Autodesk Inventor part; units mm, degrees
ref_plane "YZ Plane" through (0, 0, 0) normal (1, 0, 0) x (0, 1, 0)
ref_plane "XZ Plane" through (0, 0, 0) normal (0, 1, 0) x (-1, 0, 0)
ref_plane "XY Plane" through (0, 0, 0) normal (0, 0, 1) x (1, 0, 0)
sketch "Эскиз1" plane through (0, 0, 0) normal (0, 0, 1) x (1, 0, 0)
  line L0 (-16.05, 21) -> (16.05, 21)
  line L1 (16.05, 21) -> (16.05, -21)
  line L2 (16.05, -21) -> (-16.05, -21)
  line L3 (-16.05, -21) -> (-16.05, 21)
  point P0 (0, 0)
  point P1 (0, 21)
  point P2 (16.05, 0)
  dimension "d0" = 32.1
  dimension "d1" = 42
extrude "Выдавливание1" add sketch "Эскиз1" along normal blind 2.5
sketch "Эскиз2" plane through (0, 0, 0) normal (0, 1, 0) x (-1, 0, 0)
  line L0 (16.05, 0) -> (-16.05, 0) construction
  line L1 (16.05, 0) -> (16.05, 2.5) construction
  line L2 (-16.05, 2.5) -> (16.05, 2.5) construction
  line L3 (-16.05, 0) -> (-16.05, 2.5) construction
  line L4 (-13.75, 0) -> (-13.75, -3)
  line L5 (-13.75, -3) -> (-16.05, -3)
  line L6 (-16.05, -3) -> (-16.05, -1.8)
  line L7 (-16.05, -1.8) -> (-14.95, -1.8)
  line L8 (-14.95, -1.8) -> (-14.95, 0)
  line L9 (-14.95, 0) -> (-13.75, 0)
  line L10 (13.75, 0) -> (13.75, -3)
  line L11 (13.75, -3) -> (16.05, -3)
  line L12 (16.05, -3) -> (16.05, -1.8)
  line L13 (16.05, -1.8) -> (14.95, -1.8)
  line L14 (14.95, -1.8) -> (14.95, 0)
  line L15 (14.95, 0) -> (13.75, 0)
  point P0 (0, 0)
  dimension "d4" = 2.3
  dimension "d5" = 1.2
  dimension "d6" = 5.5
extrude "Выдавливание2" add sketch "Эскиз2" along normal mid plane 5.1
sketch "Эскиз3" plane through (0, 0, 2.5) normal (0, 0, 1) x (1, 0, 0)
  line L0 (17.05, 2.55) -> (14.95, 2.55)
  line L1 (14.95, 2.55) -> (14.95, -2.55)
  line L2 (14.95, -2.55) -> (17.05, -2.55)
  line L3 (17.05, -2.55) -> (17.05, 2.55)
  line L4 (-14.95, 2.55) -> (-17.05, 2.55)
  line L5 (-17.05, 2.55) -> (-17.05, -2.55)
  line L6 (-17.05, -2.55) -> (-14.95, -2.55)
  line L7 (-14.95, -2.55) -> (-14.95, 2.55)
  line L8 (-16.05, 21) -> (-16.05, -21) construction
  line L9 (16.05, -21) -> (16.05, 21) construction
  line L10 (16.05, -2.55) -> (16.05, 2.55) construction
  line L11 (14.95, 2.55) -> (16.05, 2.55) construction
  line L12 (14.95, -2.55) -> (14.95, 2.55) construction
  line L13 (16.05, -2.55) -> (14.95, -2.55) construction
  line L14 (-14.95, 2.55) -> (-14.95, -2.55) construction
  line L15 (-16.05, 2.55) -> (-14.95, 2.55) construction
  line L16 (-16.05, 2.55) -> (-16.05, -2.55) construction
  line L17 (-14.95, -2.55) -> (-16.05, -2.55) construction
  point P0 (0, 0)
  dimension "d9" = 1
  dimension "d10" = 1
extrude "Выдавливание3" cut sketch "Эскиз3" against normal up to surface (4.3 mm away)
sketch "Эскиз4" plane through (0, 0, 0) normal (0, 0, -1) x (-1, 0, 0)
  line L0 (13.75, -18.7) -> (-13.75, -18.7)
  line L1 (-13.75, -18.7) -> (-13.75, 18.7)
  line L2 (-13.75, 18.7) -> (13.75, 18.7)
  line L3 (13.75, 18.7) -> (13.75, -18.7)
  line L4 (-16.05, -21) -> (16.05, -21) construction
  line L5 (16.05, 21) -> (-16.05, 21) construction
  line L6 (13.75, -2.55) -> (13.75, 2.55) construction
  line L7 (-13.75, 2.55) -> (-13.75, -2.55) construction
  line L8 (16.05, -2.55) -> (16.05, -21) construction
  point P0 (0, 0)
  dimension "d13" = 2.3
  dimension "d14" = 2.3
  dimension "d15" = 2.3
extrude "Выдавливание4" cut sketch "Эскиз4" against normal blind 0.25
sketch "Эскиз5" plane through (0, 0, 2.5) normal (0, 0, 1) x (1, 0, 0)
  line L0 (14.95, 19.9) -> (-14.95, 19.9)
  line L1 (-14.95, 19.9) -> (-14.95, -19.9)
  line L2 (-14.95, -19.9) -> (14.95, -19.9)
  line L3 (14.95, -19.9) -> (14.95, 19.9)
  line L4 (14.95, -2.55) -> (14.95, 2.55) construction
  line L5 (-14.95, 2.55) -> (-14.95, -2.55) construction
  line L6 (16.05, 2.55) -> (16.05, 21) construction
  line L7 (16.05, 21) -> (-16.05, 21) construction
  line L8 (-16.05, -21) -> (16.05, -21) construction
  point P0 (0, 0)
  dimension "d18" = 1.1
  dimension "d19" = 1.1
  dimension "d20" = 1.1
extrude "Выдавливание5" cut sketch "Эскиз5" against normal blind 0.25
equation "\"d14\" = d13"
equation "\"d15\" = d13"
equation "\"d19\" = d18"
equation "\"d20\" = d18"
properties part number "D2MG cover"
Build history of the part. All positions in model axes, mm. A direction names the side the tool comes from. Round coordinates to 2 decimals unless told otherwise and drop trailing zeros. Loops run counter-clockwise (first coordinate to the right, second up) from the corner with the lowest first, then second, coordinate; pieces in that order, holes last.
Item 1: Saw through at C-C (x = -5.5). List the corners of the cut face in (y, z), then the cut area to 3 significant figures.
Item 2: Two-plate mould, pull along X, no slides. Class faces 6 (the face through (16.05, -12, 1)), 7 (the face through (-16.05, 0, -2)), 8 (the face through (13.75, 0, -1)), 9 (the face through (-15.5, 0, -1.8)): released by +X, released by -X, zero draft, split by the parting line, or undercut.
Item 3: Pin check, flat tips, straight feed: P1, Ø8, axis at x = -0.5, y = 4, coming from the +Z side; P2, Ø2.5, axis at x = 14.5, z = -1.5, coming from the +Y side; P3, Ø1.2, axis at y = -0.5, z = 1, coming from the -X side; P4, Ø2, axis at x = 9, z = -1.5, coming from the +Y side. Stop position of each tip, or through.
Item 4: Drill centre lines: line 1 along X through (y, z) = (-1, -0.9); line 2 along X through (y, z) = (-1, -2.7); line 3 along Z through (x, y) = (0, 18.5). Where is each one in solid material? Low to high.
Item 5: Which spindle directions (+Z, -Z, +X, -X, +Y, -Y) get a long thin tool onto all of the face, cutting with end or side? Do faces 1 (the face through (0, 0, 0.25)), 2 (the face through (-15.5, -2.55, 1.3)), 3 (the face through (15, -2.55, -2)), 4 (the face through (15.5, 0, -1.8)), 5 (the face through (15, 2.55, -2)). Say none if no direction does.
Item 6: Saw through at A-A (z = -2.5). List the corners of the cut face in (x, y), then the cut area to 3 significant figures.
Item 7: Saw through at B-B (y = 8.5). List the corners of the cut face in (x, z).
Worked answers:
1. outline: (-21, 0) - (-18.7, 0) - (-18.7, 0.25) - (18.7, 0.25) - (18.7, 0) - (21, 0) - (21, 2.5) - (19.9, 2.5) - (19.9, 2.25) - (-19.9, 2.25) - (-19.9, 2.5) - (-21, 2.5) - close
1. area: 85.7 mm2
2. face 6: released by +X
2. face 7: released by -X
2. face 8: undercut
2. face 9: zero draft
3. P1: stops at z = 2.25
3. P2: stops at y = 2.55
3. P3: stops at x = -14.95
3. P4: passes through
4. line 1: x = -14.95 to -13.75, 13.75 to 14.95
4. line 2: x = -16.05 to -13.75, 13.75 to 16.05
4. line 3: z = 0.25 to 2.25
5. face 1: -Z
5. face 2: +Z, -X
5. face 3: -Z, +X, -X, -Y
5. face 4: +Z, +X, +Y, -Y
5. face 5: -Z, +X, -X, +Y
6. outline: (-16.05, -2.55) - (-13.75, -2.55) - (-13.75, 2.55) - (-16.05, 2.55) - close; (13.75, -2.55) - (16.05, -2.55) - (16.05, 2.55) - (13.75, 2.55) - close
6. area: 23.5 mm2
7. outline: (-16.05, 0) - (-13.75, 0) - (-13.75, 0.25) - (13.75, 0.25) - (13.75, 0) - (16.05, 0) - (16.05, 2.5) - (14.95, 2.5) - (14.95, 2.25) - (-14.95, 2.25) - (-14.95, 2.5) - (-16.05, 2.5) - close
